Here's the drawing with two shaded views (mm, measured from the low corner). I have some questions. Round coordinates to 2 decimals unless told otherwise and drop trailing zeros. Order: outer loops, then holes, each group sorted by start corner. A loop starts at its lowest first (then second) coordinate and runs counter-clockwise, first axis right, second up. Notation, with made-up numbers: (-8.5, 17.25) -> (26.5, 17.25) arc R13 ccw to (26.5, 21.25) -> close; hole circle Ø6 at (-2.75, -7). An arc over 180 degrees is marked (long way). One line per question, with ' | ' between items.
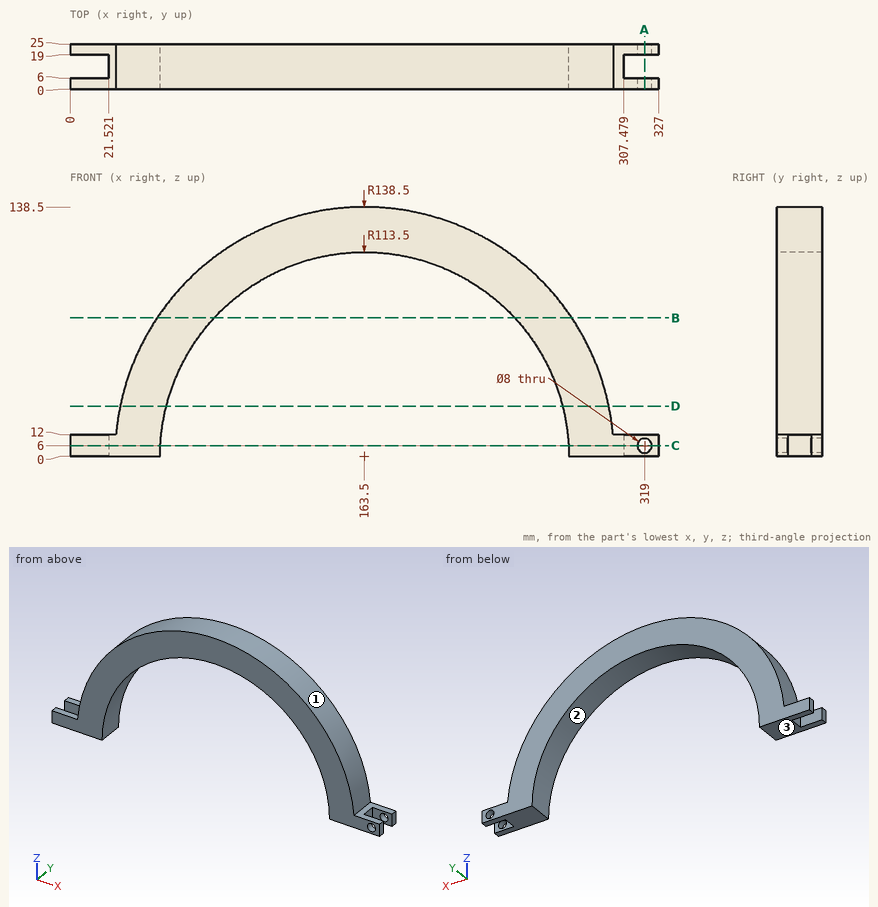
1. I want a section at D-D on z = 28. List the corners of the cut face in (x, y) for me.
From the geometry:
outline: (27.86, 0) -> (53.51, 0) -> (53.51, 25) -> (27.86, 25) -> close; (273.49, 0) -> (299.14, 0) -> (299.14, 25) -> (273.49, 25) -> close
2. I need wall thicknesses on probe 1 along Z at (x, y) = (319, 22.1); probe 2 along X at (y, z) = (18.5, 69.5); probe 3 along X at (y, z) = (2.75, 62). Which ranges of each line are inside material? Lowest first, please.
From the geometry:
probe 1: z = 0 to 2, 10 to 12 | probe 2: x = 43.7 to 73.77, 253.23 to 283.3 | probe 3: x = 39.65 to 68.43, 258.57 to 287.35
3. I want a section at C-C on z = 6. List the corners of the cut face in (x, y) for me.
From the geometry:
outline: (0, 0) -> (50.16, 0) -> (50.16, 25) -> (0, 25) -> (0, 19) -> (21.52, 19) -> (21.52, 6) -> (0, 6) -> close; (276.84, 0) -> (315, 0) -> (315, 6) -> (307.48, 6) -> (307.48, 19) -> (315, 19) -> (315, 25) -> (276.84, 25) -> close; (323, 0) -> (327, 0) -> (327, 6) -> (323, 6) -> close; (323, 19) -> (327, 19) -> (327, 25) -> (323, 25) -> close
4. If we mould it in two halves opening along X, with no side actions, what happens to the marked faces 1, 2 and 3? For each: pulls with the +X half, pulls with the -X half, needs draft (parallel to the pull), parting line crosses it, or undercut.
From the geometry:
face 1: parting line crosses it | face 2: undercut | face 3: needs draft
5. I'm going to push flat-ended pins straight in: pin 1 (2 mm diameter, centred on y = 12.5, z = 81.5, fed in from +X); pin 2 (3.5 mm diameter, centred on x = 12.5, z = 8.5, fed in from -Y); pin 3 (10 mm diameter, centred on y = 11, z = 14, fed in from -X); pin 4 (3 mm diameter, centred on x = 121.5, y = 11, fed in from +Z). Where does each tip first touch, or does it pass through?
From the geometry:
pin 1: stops at x = 276.2 | pin 2: stops at y = 0 | pin 3: stops at x = 21.52 | pin 4: stops at z = 132.45
6. I want a section at B-B on z = 77. List the corners of the cut face in (x, y) for me, and give its area (3 significant figures).
From the geometry:
outline: (48.38, 0) -> (80.11, 0) -> (80.11, 25) -> (48.38, 25) -> close; (246.89, 0) -> (278.62, 0) -> (278.62, 25) -> (246.89, 25) -> close | area: 1,590 mm²
7. I want a section at A-A on x = 319. List the corners of the cut face in (y, z) for me.
From the geometry:
outline: (0, 0) -> (6, 0) -> (6, 2) -> (0, 2) -> close; (0, 10) -> (6, 10) -> (6, 12) -> (0, 12) -> close; (19, 0) -> (25, 0) -> (25, 2) -> (19, 2) -> close; (19, 10) -> (25, 10) -> (25, 12) -> (19, 12) -> close
